Could you check a few things on this model? Use its own coordinates, in mm. Face numbers are marked on the shaded views. A direction names the side the tool comes from. Give positions to 0.01 mm unless a question says otherwise; leave off trailing zeros. Order: outer loops, then holes, each group sorted by start corner. A loop starts at its lowest first (then second) coordinate and runs counter-clockwise, first axis right, second up. Notation, with made-up numbers: M 44.25,83.5 L 96.25,83.5 A22 cw 96.25,105.5 Z; hole C 69.25,24.5 d7. An arc over 180 degrees is marked long. Use a Markdown table: item, result. Add a question column.
```python
from build123d import *

# Parameters (mm, degrees)
F0_R      = 3.5
F1_DEPTH  = 15
F5_DEPTH  = 23
F6_DEPTH  = 19
F2_R      = 3.5
F7_DEPTH  = 26
F8_DEPTH  = 2.5
F12_DEPTH = 19
F13_DEPTH = 23
F14_DEPTH = 2.5
F15_DEPTH = 25.1
F16_R     = 2.5
F17_DEPTH = 25


with BuildPart() as f1:
    # F0 (on Front) → F1 (new body)
    with BuildSketch(Plane.XZ):
        Polygon((36, 10), (-36, 10), (-36, 0), (-36, -10), (36, -10), (36, 0), (36, 7.5), align=None)
        with Locations((-21, 0)):
            Circle(F0_R, mode=Mode.SUBTRACT)
        with Locations((21, 0)):
            Circle(F0_R, mode=Mode.SUBTRACT)
        Polygon((-36, 0), (-36, 10), (-47.5, 0), align=None)
        Polygon((38.875, 7.5), (36, 10), (36, 7.5), align=None)
        Polygon((66, 10), (36, 10), (38.875, 7.5), (66, 7.5), align=None)
        Polygon((-36, -10), (-36, 0), (-47.5, 0), (-59, 0), (-59, -10), align=None)
        Polygon((38.875, 7.5), (36, 7.5), (36, 0), (47.5, 0), align=None)
        Polygon((-36, -25), (-36, -10), (-59, -10), (-59, -25.0883084536), align=None)
        Polygon((47.5, 0), (36, 0), (36, -10), (36, -25), (59, -25.0883084536), (59, -10), (59, 0), align=None)
    extrude(amount=F1_DEPTH)

    # F3 (on face) → F5 (cut)
    with BuildSketch(Plane.YZ.offset(59)):
        with BuildLine():
            ThreePointArc((-5.75, -18.0883084536), (-8.7374368671, -16.8508715865), (-7.5, -19.8383084536))
            ThreePointArc((-7.5, -19.8383084536), (-6.2625631329, -19.3257453206), (-5.75, -18.0883084536))
        make_face()
    extrude(amount=-F5_DEPTH, mode=Mode.SUBTRACT)

    # F3 (on face) → F6 (cut)
    with BuildSketch(Plane.YZ.offset(59)):
        with BuildLine():
            ThreePointArc((-4.5, -18.0883084536), (-9.6213203436, -15.96698811), (-7.5, -21.0883084536))
            ThreePointArc((-7.5, -21.0883084536), (-5.3786796564, -20.2096287971), (-4.5, -18.0883084536))
        make_face()
        with BuildLine():
            ThreePointArc((-5.75, -18.0883084536), (-6.2625631329, -19.3257453206), (-7.5, -19.8383084536))
            ThreePointArc((-7.5, -19.8383084536), (-8.7374368671, -16.8508715865), (-5.75, -18.0883084536))
        make_face(mode=Mode.SUBTRACT)
    extrude(amount=-F6_DEPTH, mode=Mode.SUBTRACT)

    # F2 (on face) → F7 (cut)
    with BuildSketch(Plane(origin=(-0.0954553395, 0, -24.8614115721), x_dir=(0.9999926292, 0, -0.0038394697), z_dir=(-0.0038394697, 0, -0.9999926292))):
        with Locations((54.095890923, 7.5)):
            Circle(F2_R)
    extrude(amount=-F7_DEPTH, mode=Mode.SUBTRACT)

    # F4 (on face) → F8 (cut)
    with BuildSketch(Plane(origin=(36, 0, 0), x_dir=(0, -1, 0), z_dir=(-1, 0, 0))):
        Polygon((4.675, -20.825), (7.5, -20.825), (10.325, -20.825), (10.325, -15.175), (4.675, -15.175), align=None)
    extrude(amount=-F8_DEPTH, mode=Mode.SUBTRACT)

    # F9 (on face) → F12 (cut)
    with BuildSketch(Plane(origin=(-59, 0, 0), x_dir=(0, -1, 0), z_dir=(-1, 0, 0))):
        with BuildLine():
            ThreePointArc((10.5, -18.0883084536), (5.3786796564, -15.96698811), (7.5, -21.0883084536))
            ThreePointArc((7.5, -21.0883084536), (9.6213203436, -20.2096287971), (10.5, -18.0883084536))
        make_face()
        with BuildLine():
            ThreePointArc((9.25, -18.0883084536), (8.7374368671, -19.3257453206), (7.5, -19.8383084536))
            ThreePointArc((7.5, -19.8383084536), (6.2625631329, -16.8508715865), (9.25, -18.0883084536))
        make_face(mode=Mode.SUBTRACT)
    extrude(amount=-F12_DEPTH, mode=Mode.SUBTRACT)

    # F9 (on face) → F13 (cut)
    with BuildSketch(Plane(origin=(-59, 0, 0), x_dir=(0, -1, 0), z_dir=(-1, 0, 0))):
        with BuildLine():
            ThreePointArc((9.25, -18.0883084536), (6.2625631329, -16.8508715865), (7.5, -19.8383084536))
            ThreePointArc((7.5, -19.8383084536), (8.7374368671, -19.3257453206), (9.25, -18.0883084536))
        make_face()
    extrude(amount=-F13_DEPTH, mode=Mode.SUBTRACT)

    # F10 (on face) → F14 (cut)
    with BuildSketch(Plane.YZ.offset(-36)):
        Polygon((-10.325, -20.825), (-7.5, -20.825), (-4.675, -20.825), (-4.675, -15.175), (-10.325, -15.175), align=None)
    extrude(amount=-F14_DEPTH, mode=Mode.SUBTRACT)

    # F11 (on face) → F15 (cut)
    with BuildSketch(Plane(origin=(0.0954553395, 0, -24.8614115721), x_dir=(0.9999926292, 0, 0.0038394697), z_dir=(0.0038394697, 0, -0.9999926292))):
        with BuildLine():
            ThreePointArc((-50.595890923, 7.5), (-54.095890923, 11), (-57.595890923, 7.5))
            ThreePointArc((-57.595890923, 7.5), (-54.095890923, 4), (-50.595890923, 7.5))
        make_face()
    extrude(amount=-F15_DEPTH, mode=Mode.SUBTRACT)

    # F16 (on face) → F17 (cut)
    with BuildSketch(Plane(origin=(0, 0, 7.5), x_dir=(1, 0, 0), z_dir=(0, 0, -1))):
        with Locations((61, 7.5)):
            Circle(F16_R)
    extrude(amount=-F17_DEPTH, mode=Mode.SUBTRACT)


solid = f1.part
```
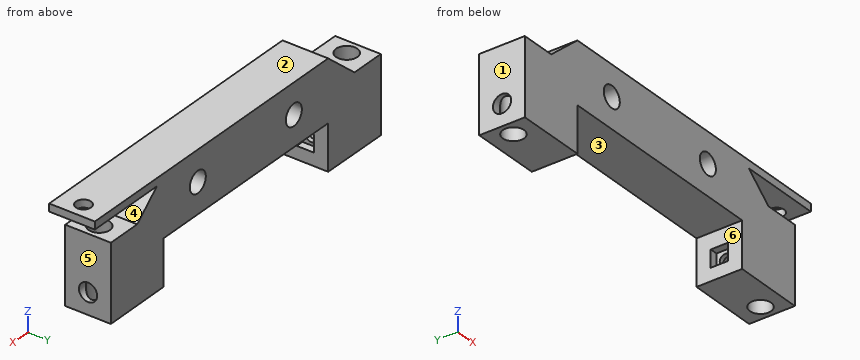
1) For pin 1 (2 mm diameter, centred on x = 37, y = -7, fed in from -Z); pin 2 (4 mm diameter, centred on y = -8.5, z = -11, fed in from +X); pin 3 (1.8 mm diameter, centred on y = -8, z = -18, fed in from -X); pin 4 (1 mm diameter, centred on x = 2, y = -5, fed in from -Z), each with a flat end and sliding along its axis, tell me the tip position at first contact or that it passes through.
2) Suppose I cut it at C-C on z = -12.5. Count the separate pieces of the cut face and the enclosed holes in it, and give its area (3 significant figures).
3) Suppose I cut it at D-D on x = 8. Please give me the cut outline in (y, z), and give its area (3 significant figures).
4) Suppose I cut it at B-B on x = 61. Please give me the cut outline in (y, z).
5) We'd pull the mould along X, two halves only. Please class the marked faces 1, 2 and 3: pulls with the +X half, pulls with the -X half, needs draft (parallel to the pull), parting line crosses it, or undercut.
6) Please list where these lines run through material, in increasing order: line 1 (X direction, y = -4.5, z = -12.5); line 2 (X direction, y = -12.25, z = -18); line 3 (Z direction, x = -28.5, y = -8.5). Write a range as from..to.
7) Suppose I cut it at A-A on y = -13.25. Please give me the cut outline in (x, z) (3 decimals).
8) For the marked faces 4, 5 and 6, which set-ups out of +Z, -Z, +X, -X, +Y, -Y let a thin tool reach every point of the face, with its end or its side?
Values found:
| question | item | result |
|---|---|---|
| 1 | pin 1 | stops at z = -25.01 |
| 1 | pin 2 | stops at x = 59 |
| 1 | pin 3 | passes through |
| 1 | pin 4 | stops at z = -10 |
| 2 | separate pieces | 2 |
| 2 | enclosed holes | 2 |
| 2 | area | 613 mm^2 |
| 3 | outline | M -15,-10 L 0,-10 L 0,10 L -15,10 Z |
| 3 | area | 300 mm^2 |
| 4 | outline | M -15,7.5 L -10,7.5 L -10,10 L -15,10 Z; M -5,7.5 L 0,7.5 L 0,10 L -5,10 Z |
| 5 | face 1 | pulls with the -X half |
| 5 | face 2 | needs draft |
| 5 | face 3 | undercut |
| 6 | line 1 | x = -59..-55.85, -52.25..-36, 36..52.25, 55.85..59 |
| 6 | line 2 | x = -59..-36, 36..59 |
| 6 | line 3 | z = -10..10 |
| 7 | outline | M -59,-25.088 L -36,-25 L -36,-10 L 36,-10 L 36,-25 L 59,-25.088 L 59,0 L 47.5,0 L 38.875,7.5 L 66,7.5 L 66,10 L -36,10 L -47.5,0 L -59,0 Z; hole C -21,0 d7; hole C 21,0 d7 |
| 8 | face 4 | +X, +Y, -Y |
| 8 | face 5 | -Z, +X, +Y, -Y |
| 8 | face 6 | -Z, +Y, -Y |
